```python
from build123d import *

# Parameters (mm, degrees)
F0_R     = 6.875
F1_DEPTH = 40
F0_W     = 60
F0_H     = 80
F2_DEPTH = 20
F3_R     = 19.25
F3_R_2   = 9.5
F4_DEPTH = 3.5
F5_W     = 60
F5_H     = 40
F6_DEPTH = 50


with BuildPart() as f1:
    # F0 (on Front) → F1 (new body)
    with BuildSketch(Plane.XZ):
        with Locations((0, 40)):
            Circle(F0_R)
    extrude(amount=F1_DEPTH)

    # F0 (on Front) → F2 (join)
    with BuildSketch(Plane.XZ):
        with Locations((0, 40)):
            Rectangle(F0_W, F0_H)
        with Locations((0, 40)):
            Circle(F0_R, mode=Mode.SUBTRACT)
        with Locations((0, 40)):
            Circle(F0_R)
    extrude(amount=-F2_DEPTH)

    # F3 (on face) → F4 (cut)
    with BuildSketch(Plane.XZ):
        with Locations((0, 40)):
            Circle(F3_R)
        with Locations((0, 40)):
            Circle(F3_R_2, mode=Mode.SUBTRACT)
    extrude(amount=-F4_DEPTH, mode=Mode.SUBTRACT)

    # F5 (on face) → F6 (join)
    with BuildSketch(Plane(origin=(0, 20, 0), x_dir=(-1, 0, 0), z_dir=(0, 1, 0))):
        with Locations((0, 20)):
            Rectangle(F5_W, F5_H)
    extrude(amount=F6_DEPTH)


solid = f1.part
```
The listing builds one solid part. Answer for the finished solid, in the listing's coordinates (mm). A direction names the side the tool comes from. Coordinates: 2 decimals unless noted, no trailing zeros. Loops run counter-clockwise (first coordinate to the right, second up) from the corner with the lowest first, then second, coordinate; pieces in that order, holes last. Notation, with made-up numbers: (26.25, -31) - (54.25, -31) arc R37 ccw to (54.25, 8) - close; hole circle Ø8 at (41, 1.25). An arc over 180 degrees is marked (long way). Use a Markdown table: item, result. Add a question column.
1) The part is cut by section B-B, the plane z = 27.5. Give the vertices of the cut face in (x, y).
2) Find the intervals of material crossed by line 1 (Z direction, x = 0, y = 2); line 2 (Z direction, x = -28, y = 47); line 3 (Y direction, x = 10, z = 39), in increasing order.
3) The part is cut by section A-A, the plane x = 0. Give the vertices of the cut face in (y, z) (3 decimals), and give its area (3 significant figures).
4) The part is cut by section C-C, the plane y = 26.5. Give the vertices of the cut face in (x, z).
5) The mould has two halves that part along X. Classify faces 1 (the flat face through (0, -40, 40)), 2 (the cylindrical face through (-1.24, 1.73, 49.42)), 3 (the cylindrical face through (-4.173, 1.726, 21.208)), 4 (the flat face through (30, 27, 31)): released by +X, released by -X, zero draft, split by the parting line, or undercut.
6) For faces 5 (the flat face through (0, 35, 0)), 6 (the cylindrical face through (6.558, -19.72, 42.065)), 7 (the flat face through (0, 45, 40)), determine the directions among +Z, -Z, +X, -X, +Y, -Y from which every point of the face is accessible in a straight line to the end or side of a thin tool.
7) Given pin 1 (25 mm diameter, centred on x = 0.5, y = 54.5, fed in from +Z); pin 2 (3 mm diameter, centred on x = 22.5, z = 48.5, fed in from +Y); pin 3 (4 mm diameter, centred on x = -1, y = -18.5, fed in from -Z) (3 decimals), each flat-ended and moving along its own axis, determine where each tip first touches the part or whether it passes through.
8) The part is cut by section D-D, the plane x = -17.5. Give the vertices of the cut face in (y, z), and give its area (3 significant figures).
Here are the results:
| question | item | result |
|---|---|---|
| 1 | outline | (-30, 0) - (-14.64, 0) - (-14.64, 3.5) - (14.64, 3.5) - (14.64, 0) - (30, 0) - (30, 70) - (-30, 70) - close |
| 2 | line 1 | z = 0 to 20.75, 30.5 to 49.5, 59.25 to 80 |
| 2 | line 2 | z = 0 to 40 |
| 2 | line 3 | y = 3.5 to 70 |
| 3 | outline | (-40, 33.125) - (0, 33.125) - (0, 30.5) - (3.5, 30.5) - (3.5, 20.75) - (0, 20.75) - (0, 0) - (70, 0) - (70, 40) - (20, 40) - (20, 80) - (0, 80) - (0, 59.25) - (3.5, 59.25) - (3.5, 49.5) - (0, 49.5) - (0, 46.875) - (-40, 46.875) - close |
| 3 | area | 4,080 mm^2 |
| 4 | outline | (-30, 0) - (30, 0) - (30, 40) - (-30, 40) - close |
| 5 | face 1 | zero draft |
| 5 | face 2 | undercut |
| 5 | face 3 | undercut |
| 5 | face 4 | released by +X |
| 6 | face 5 | -Z, +X, -X, +Y, -Y |
| 6 | face 6 | -Y |
| 6 | face 7 | +Z, +X, -X, +Y |
| 7 | pin 1 | stops at z = 40 |
| 7 | pin 2 | stops at y = 20 |
| 7 | pin 3 | stops at z = 33.125 |
| 8 | outline | (0, 0) - (70, 0) - (70, 40) - (20, 40) - (20, 80) - (0, 80) - (0, 48.02) - (3.5, 48.02) - (3.5, 31.98) - (0, 31.98) - close |
| 8 | area | 3,540 mm^2 |
